Model file for the job. Use its own axes, mm. A direction names the side the tool comes from. Round coordinates to 2 decimals unless told otherwise and drop trailing zeros. Order: outer loops, then holes, each group sorted by start corner. A loop starts at its lowest first (then second) coordinate and runs counter-clockwise, first axis right, second up. Notation, with made-up numbers: M 37.25,8 L 48.25,8 A16 ccw 48.25,27 Z; hole C 39.5,36.5 d1. An arc over 180 degrees is marked long. Return JSON: item names as keys, results as strings. Group by question number.
Item 1: Probe line 1 along Y through (x, z) = (0, -9.25) (3 decimals); line 2 along X through (y, z) = (2.1, -12); line 3 along X through (y, z) = (0.9, -3.5). List the from-to ranges inside material, lowest first.
Item 2: Slice it at B-B on z = -4.5. Write the cut outline in (x, y), then the cut area to 3 significant figures.
Item 3: Which spindle directions (+Z, -Z, +X, -X, +Y, -Y) get a long thin tool onto all of the face, cutting with end or side? Do faces 5 (the face through (-4.927, 1.892, -12.16)), 6 (the face through (-3.16, 1.88, -11.8)), 7 (the face through (-1, 3, -6.35)). Say none if no direction does.
Item 4: Pull direction X, two halves, no side cores. Call faces 1 (the face through (0.22, 0.93, -9.57)), 2 (the face through (38.1, 2, -6)), 3 (the face through (19, 0, -6)), 4 (the face through (-3.165, 3.161, -9.569)): pulls with the +X half, pulls with the -X half, needs draft (parallel to the pull), parting line crosses it, or undercut.
Item 5: Pin check, flat tips, straight feed: pin 1 Ø0.6 at (x, y) = (-4.5, 1.5) entering from -Z; pin 2 Ø1.1 at (x, y) = (-2, 2) entering from +Z; pin 3 Ø2 at (y, z) = (2.5, -4.5) entering from -X. Stop position of each tip, or through.
Item 6: Slice it at A-A on z = -8. Write the cut outline in (x, y) (3 decimals).
from build123d import *

# Parameters (mm, degrees)
SKETCH1_W           = 38.1
SKETCH1_H           = 12.7
BOSS_EXTRUDE1_DEPTH = 3.81
SKETCH2_W           = 4.064
SKETCH2_H           = 6.35
CUT_EXTRUDE1_DEPTH  = 4.81
SKETCH4_R           = 1
CUT_EXTRUDE2_DEPTH  = 13.7
SKETCH5_R           = 1
BOSS_EXTRUDE2_DEPTH = 6.35
CUT_EXTRUDE3_DEPTH  = 4.81
FILLET1_R           = 0.508


with BuildPart() as part:
    # Sketch1 → Boss-Extrude1 (new body)
    with BuildSketch(Plane(origin=(0, 0, 0), x_dir=(1, 0, 0), z_dir=(0, 1, 0))):
        with Locations((19.05, 6.35)):
            Rectangle(SKETCH1_W, SKETCH1_H)
    extrude(amount=BOSS_EXTRUDE1_DEPTH)

    # Sketch2 → Cut-Extrude1 (cut, through all)
    with BuildSketch(Plane(origin=(0, 3.81, 0), x_dir=(1, 0, 0), z_dir=(0, 1, 0))):
        with Locations((2.032, 3.175)):
            Rectangle(SKETCH2_W, SKETCH2_H)
    extrude(amount=-CUT_EXTRUDE1_DEPTH, mode=Mode.SUBTRACT)

    # Sketch4 → Cut-Extrude2 (cut, through all)
    with BuildSketch(Plane(origin=(0, 0, -12.7), x_dir=(-1, 0, 0), z_dir=(0, 0, -1))):
        with Locations((0, 1.905)):
            Circle(SKETCH4_R)
    extrude(amount=-CUT_EXTRUDE2_DEPTH, mode=Mode.SUBTRACT)

    # Sketch5 → Boss-Extrude2 (add)
    with BuildSketch(Plane(origin=(0, 0, -12.7), x_dir=(-1, 0, 0), z_dir=(0, 0, -1))):
        with BuildLine():
            Line((0.407900981, 3.765817506), (6, 2.54))
            Line((6, 2.54), (6, 1.27))
            Line((6, 1.27), (0.407900981, 0.044182494))
            ThreePointArc((0.407900981, 0.044182494), (-1.905, 1.905), (0.407900981, 3.765817506))
        make_face()
        with Locations((0, 1.905)):
            Circle(SKETCH5_R, mode=Mode.SUBTRACT)
    extrude(amount=-BOSS_EXTRUDE2_DEPTH)

    # Sketch6 → Cut-Extrude3 (cut, through all)
    with BuildSketch(Plane.XZ):
        Polygon((-4.73, -12.7), (-5.377139077, -10.922), (-4.107139077, -10.922), (-2.19, -12.7), align=None)
    extrude(amount=-CUT_EXTRUDE3_DEPTH, mode=Mode.SUBTRACT)

    # Fillet1
    fillet1_edges = [part.edges().sort_by_distance(p)[0] for p in [
        (-5.377139077, 1.905, -10.922),
    ]]
    fillet(fillet1_edges, radius=FILLET1_R)


solid = part.part
Output values:
{
 "1": {"line 1": "0 to 0.905, 2.905 to 3.81", "line 2": "-6 to -4.98, -2.94 to -0.98, 0.98 to 38.1", "line 3": "4.06 to 38.1"},
 "2": {"outline": "M 4.06,0 L 38.1,0 L 38.1,3.81 L 4.06,3.81 Z", "area": "130 mm²"},
 "3": {"face 5": "+Y, -Y", "face 6": "-Z, +Y, -Y", "face 7": "+Z, -X, +Y, -Y"},
 "4": {"face 1": "undercut", "face 2": "pulls with the +X half", "face 3": "needs draft", "face 4": "pulls with the -X half"},
 "5": {"pin 1": "z = -12.7", "pin 2": "z = -6.35", "pin 3": "x = 4.06"},
 "6": {"outline": "M -6,1.27 L -0.408,0.044 A1.905 ccw 0,0 L 38.1,0 L 38.1,3.81 L 0,3.81 A1.905 ccw -0.408,3.766 L -6,2.54 Z; hole C 0,1.905 d2"}
}
